Source: CAD feature listing. Evaluate the final solid. Frame: model axes, mm. A direction names the side the tool comes from. Give positions to 0.01 mm unless a question says otherwise; leave off trailing zeros. Order: outer loops, then holes, each group sorted by start corner. A loop starts at its lowest first (then second) coordinate and runs counter-clockwise, first axis right, second up.
from build123d import *

# Parameters (mm, degrees)
F0_R          = 1.1303
F0_R_2        = 3.556
F1_DEPTH      = 3.96875
F2_R          = 7.9375
F2_R_2        = 3.556
F3_DEPTH      = 3.175
F3_DEPTH_BACK = 20.6375
F5_DEPTH      = 4.445
F6_R          = 1.143
F7_DEPTH      = 20.0161085099
F8_R          = 1.143
F9_DEPTH      = 23.1380417346


with BuildPart() as f1:
    # F0 (on Front) → F1 (new body)
    with BuildSketch(Plane.XZ):
        with BuildLine():
            ThreePointArc((-7.6823660714, -1.9962860002), (-7.9375, 0), (-7.6823660714, 1.9962860002))
            ThreePointArc((-7.6823660714, 1.9962860002), (-9.7917396627, 3.7425350625), (-12.5299107143, 3.707010039))
            ThreePointArc((-12.5299107143, 3.707010039), (-15.08125, 0), (-12.5299107143, -3.707010039))
            ThreePointArc((-12.5299107143, -3.707010039), (-9.7917396627, -3.7425350625), (-7.6823660714, -1.9962860002))
        make_face()
        with Locations((-11.1125, 0)):
            Circle(F0_R, mode=Mode.SUBTRACT)
        with BuildLine():
            ThreePointArc((12.5299107143, 3.707010039), (9.7917396627, 3.7425350625), (7.6823660714, 1.9962860002))
            ThreePointArc((7.6823660714, 1.9962860002), (7.8734581647, 1.0062617845), (7.9375, 0))
            ThreePointArc((7.9375, 0), (7.8734581647, -1.0062617845), (7.6823660714, -1.9962860002))
            ThreePointArc((7.6823660714, -1.9962860002), (9.7917396627, -3.7425350625), (12.5299107143, -3.707010039))
            ThreePointArc((12.5299107143, -3.707010039), (14.381775557, -2.2500697534), (15.08125, 0))
            ThreePointArc((15.08125, 0), (14.381775557, 2.2500697534), (12.5299107143, 3.707010039))
        make_face()
        with Locations((11.1125, 0)):
            Circle(F0_R, mode=Mode.SUBTRACT)
        with BuildLine():
            ThreePointArc((7.6823660714, 1.9962860002), (5.9152995581, 5.292743843), (2.8348214286, 7.4140200781))
            ThreePointArc((2.8348214286, 7.4140200781), (0, 7.9375), (-2.8348214286, 7.4140200781))
            ThreePointArc((-2.8348214286, 7.4140200781), (-5.9152995581, 5.292743843), (-7.6823660714, 1.9962860002))
            ThreePointArc((-7.6823660714, 1.9962860002), (-7.2807692819, 1.0338357059), (-7.14375, 0))
            ThreePointArc((-7.14375, 0), (-7.2807692819, -1.0338357059), (-7.6823660714, -1.9962860002))
            ThreePointArc((-7.6823660714, -1.9962860002), (-5.9152995581, -5.292743843), (-2.8348214286, -7.4140200781))
            ThreePointArc((-2.8348214286, -7.4140200781), (0, -7.9375), (2.8348214286, -7.4140200781))
            ThreePointArc((2.8348214286, -7.4140200781), (5.9152995581, -5.292743843), (7.6823660714, -1.9962860002))
            ThreePointArc((7.6823660714, -1.9962860002), (7.14375, 0), (7.6823660714, 1.9962860002))
        make_face()
        Circle(F0_R_2, mode=Mode.SUBTRACT)
        with BuildLine():
            ThreePointArc((-7.14375, 0), (-7.2807692819, 1.0338357059), (-7.6823660714, 1.9962860002))
            ThreePointArc((-7.6823660714, 1.9962860002), (-7.9375, 0), (-7.6823660714, -1.9962860002))
            ThreePointArc((-7.6823660714, -1.9962860002), (-7.2807692819, -1.0338357059), (-7.14375, 0))
        make_face()
        with BuildLine():
            ThreePointArc((7.9375, 0), (7.8734581647, 1.0062617845), (7.6823660714, 1.9962860002))
            ThreePointArc((7.6823660714, 1.9962860002), (7.14375, 0), (7.6823660714, -1.9962860002))
            ThreePointArc((7.6823660714, -1.9962860002), (7.8734581647, -1.0062617845), (7.9375, 0))
        make_face()
        with BuildLine():
            Line((12.5299107143, 3.707010039), (2.8348214286, 7.4140200781))
            ThreePointArc((2.8348214286, 7.4140200781), (5.9152995581, 5.292743843), (7.6823660714, 1.9962860002))
            ThreePointArc((7.6823660714, 1.9962860002), (9.7917396627, 3.7425350625), (12.5299107143, 3.707010039))
        make_face()
        with BuildLine():
            ThreePointArc((-7.6823660714, 1.9962860002), (-5.9152995581, 5.292743843), (-2.8348214286, 7.4140200781))
            Line((-2.8348214286, 7.4140200781), (-12.5299107143, 3.707010039))
            ThreePointArc((-12.5299107143, 3.707010039), (-9.7917396627, 3.7425350625), (-7.6823660714, 1.9962860002))
        make_face()
        with BuildLine():
            ThreePointArc((-2.8348214286, -7.4140200781), (-5.9152995581, -5.292743843), (-7.6823660714, -1.9962860002))
            ThreePointArc((-7.6823660714, -1.9962860002), (-9.7917396627, -3.7425350625), (-12.5299107143, -3.707010039))
            Line((-12.5299107143, -3.707010039), (-2.8348214286, -7.4140200781))
        make_face()
        with BuildLine():
            ThreePointArc((12.5299107143, -3.707010039), (9.7917396627, -3.7425350625), (7.6823660714, -1.9962860002))
            ThreePointArc((7.6823660714, -1.9962860002), (5.9152995581, -5.292743843), (2.8348214286, -7.4140200781))
            Line((2.8348214286, -7.4140200781), (12.5299107143, -3.707010039))
        make_face()
    extrude(amount=F1_DEPTH)

    # F2 (on face) → F3 (join, two sides)
    with BuildSketch(Plane.XZ.offset(3.96875)) as f3_sk:
        Circle(F2_R)
        Circle(F2_R_2, mode=Mode.SUBTRACT)
    extrude(amount=F3_DEPTH)
    extrude(f3_sk.sketch, amount=-F3_DEPTH_BACK)

    # F4 (on face) → F5 (join)
    with BuildSketch(Plane(origin=(0, 16.66875, 0), x_dir=(-1, 0, 0), z_dir=(0, 1, 0))):
        Polygon((-4.6868976554, 3.8834653813), (-2.5368989125, 4.9789444572), (-0.3869001697, 6.074423533), (-0.6175273435, 6.5270548473), (-4.9175248293, 4.3360966956), align=None)
        Polygon((-6.074423533, -0.3869001697), (-6.5270548473, -0.6175273435), (-4.3360966956, -4.9175248293), (-3.8834653813, -4.6868976554), (-4.9789444572, -2.5368989125), align=None)
        Polygon((0.3869001697, -6.074423533), (0.6175273435, -6.5270548473), (4.9175248293, -4.3360966956), (4.6868976554, -3.8834653813), (2.5368989125, -4.9789444572), align=None)
        Polygon((6.074423533, 0.3869001697), (6.5270548473, 0.6175273435), (4.3360966956, 4.9175248293), (3.8834653813, 4.6868976554), (4.9789444572, 2.5368989125), align=None)
    extrude(amount=F5_DEPTH)

    # F6 (on face) → F7 (cut, through all)
    with BuildSketch(Plane(origin=(2.7675260864, 0, 5.4315757715), x_dir=(0.8910065242, 0, -0.4539904997), z_dir=(0.4539904997, 0, 0.8910065242))):
        with BuildLine():
            Line((-2.413, 21.11375), (-2.413, 18.82775))
            ThreePointArc((-2.413, 18.82775), (-1.7434461018, 20.4441961018), (-0.127, 21.11375))
            Line((-0.127, 21.11375), (-2.413, 21.11375))
        make_face()
        with Locations((0, 18.82775)):
            Circle(F6_R)
        with BuildLine():
            ThreePointArc((0.127, 21.11375), (1.7434461018, 20.4441961018), (2.413, 18.82775))
            Line((2.413, 18.82775), (2.413, 21.11375))
            Line((2.413, 21.11375), (0.127, 21.11375))
        make_face()
    extrude(amount=-F7_DEPTH, mode=Mode.SUBTRACT)

    # F8 (on face) → F9 (cut, through all)
    with BuildSketch(Plane(origin=(5.4315757715, 0, -2.7675260864), x_dir=(0, 1, 0), z_dir=(0.8910065242, 0, -0.4539904997))):
        with BuildLine():
            Line((21.11375, 0.127), (21.11375, 2.413))
            Line((21.11375, 2.413), (18.82775, 2.413))
            ThreePointArc((18.82775, 2.413), (20.4441961018, 1.7434461018), (21.11375, 0.127))
        make_face()
        with Locations((18.82775, 0)):
            Circle(F8_R)
        with BuildLine():
            Line((21.11375, -2.413), (21.11375, -0.127))
            ThreePointArc((21.11375, -0.127), (20.4441961018, -1.7434461018), (18.82775, -2.413))
            Line((18.82775, -2.413), (21.11375, -2.413))
        make_face()
    extrude(amount=-F9_DEPTH, mode=Mode.SUBTRACT)


solid = f1.part
1) Reachability of faces 1 (the face through (-5.447, 17.378, 2.737)), 2 (the face through (10.279, -1.957, 0.764)), 3 (the face through (-2.737, 17.378, -5.447)) from +Z, -Z, +X, -X, +Y, -Y: full face, straight path, thin tool, end or side. Return the list, or none.
Checks:
face 1: +Z, -X, +Y
face 2: +Y, -Y
face 3: -Z, -X, +Y
2) Section query B-B on y = 13. Output: boundary loops of the cut face in (x, z) (1 decimal), and give its area (3 significant figures).
Checks:
outline: circle Ø15.9 at (0, 0); hole circle Ø7.1 at (0, 0)
area: 158 mm2
3) Ray query, L1, parallel to Z at x = 0, y = -2.85; L2, parallel to Y at x = -11, z = 4; L3, parallel to X at y = 1, z = -0.75. Return the intervals inside material, ascending.
Checks:
L1: z = -7.94 to -3.56, 3.56 to 7.94
L2: y = -3.97 to 0
L3: x = -7.9 to -3.48, 3.48 to 7.9
4) First-contact query: pin 1 Ø5.5 at (x, z) = (0, 0) entering from -Y (3 decimals); pin 2 Ø4 at (x, y) = (-5, -3.5) entering from +Z; pin 3 Ø1.5 at (y, z) = (18, 5.5) entering from +X; pin 4 Ø4 at (y, z) = (15.5, 2) entering from +X. Flat tips, straight axial feed; report the tip coordinate or a pass-through.
Checks:
pin 1: passes through
pin 2: stops at z = 7.35
pin 3: stops at x = 4.11
pin 4: stops at x = 7.94
5) Pull-direction query (Z, two-part tool) for faces 4 (the face through (-4.22, 20.426, -4.403)), 5 (the face through (4.425, 20.462, -4.191)), 6 (the face through (-4.403, 20.426, 4.22)); classes: +Z half, -Z half, draft (parallel to the pull), parting line (faces both ways), or undercut.
Checks:
face 4: undercut
face 5: -Z half
face 6: +Z half
6) Section query A-A on x = 0. Output: boundary loops of the cut face in (y, z).
Checks:
outline: (-7.14, -7.94) - (16.67, -7.94) - (16.67, -3.56) - (-7.14, -3.56) - close; (-7.14, 3.56) - (16.67, 3.56) - (16.67, 7.94) - (-7.14, 7.94) - close
